from build123d import *

# Parameters (mm, degrees)
BOSS_EXTRUDE1_DEPTH     = 3
HOLE2_AT_2_COUNT        = 2
HOLE2_AT_2_PITCH        = 6
HOLE2_AT_3_COUNT        = 2
HOLE2_AT_3_PITCH        = 12
HOLE3_OUTLINE_R         = 2.5
HOLE3_DEPTH             = 1.5
SKETCH8_R               = 2.5
CUT_EXTRUDE1_DEPTH      = 1
FILL_START              = 2
FILL_PATTERN2_OUTLINE_R = 2.5
FILL_PATTERN2_DEPTH     = 1
HOLE6_D                 = 4
HOLE6_DEPTH             = 1.5
HOLE6_CBORE_D           = 5
HOLE6_CBORE_DEPTH       = 1
HOLE6_TIP               = 1.201721238
HOLE7_D                 = 4
HOLE7_DEPTH             = 3
HOLE7_CBORE_D           = 5
HOLE7_CBORE_DEPTH       = 1
HOLE7_TIP               = 1.201721238
HOLE8_D                 = 2
HOLE8_DEPTH             = 3
HOLE8_CBORE_D           = 3.8
HOLE8_CBORE_DEPTH       = 1.5
HOLE8_TIP               = 0.600860619


# Read off the part's stored shape, not the designer's step: Hole3, Fill Pattern2
with BuildPart() as part:
    # Sketch1 → Boss-Extrude1 (new body)
    with BuildSketch(Plane(origin=(0, 0, 0), x_dir=(1, 0, 0), z_dir=(0, 1, 0))):
        with BuildLine():
            Line((-12, 9), (12, 9))
            ThreePointArc((12, 9), (14.121320344, 8.121320344), (15, 6))
            Line((15, 6), (15, -6))
            ThreePointArc((15, -6), (14.121320344, -8.121320344), (12, -9))
            Line((12, -9), (-12, -9))
            ThreePointArc((-12, -9), (-14.121320344, -8.121320344), (-15, -6))
            Line((-15, -6), (-15, 6))
            ThreePointArc((-15, 6), (-14.121320344, 8.121320344), (-12, 9))
        make_face()
    extrude(amount=BOSS_EXTRUDE1_DEPTH)

    # Sketch3 → Hole2 (revolve, cut)
    with BuildSketch(Plane(origin=(-11.5, 3, -6), x_dir=(0, 0, 1), z_dir=(1, 0, 0))):
        Polygon((0, 0), (0, 2.701721238), (2, 1.5), (2, 0.8), (2.5, 0.8), (2.5, 0), align=None)
    hole2 = revolve(axis=Axis((-11.5, 14.310875039, -6), (0, -1, 0)), mode=Mode.SUBTRACT)

    # Hole2 at 2: Hole2 ×2
    with Locations(*[(0, 0, i * HOLE2_AT_2_PITCH) for i in range(1, HOLE2_AT_2_COUNT)]):
        add(hole2, mode=Mode.SUBTRACT)

    # Hole2 at 3: Hole2 ×2
    with Locations(*[(0, 0, i * HOLE2_AT_3_PITCH) for i in range(1, HOLE2_AT_3_COUNT)]):
        add(hole2, mode=Mode.SUBTRACT)

    # Hole3 outline → Hole3 (cut)
    with BuildSketch(Plane(origin=(0, 0, 0), x_dir=(1, 0, 0), z_dir=(0, 1, 0))):
        with Locations((-11.5, -6)):
            Circle(HOLE3_OUTLINE_R)
        with Locations((-11.5, 0)):
            Circle(HOLE3_OUTLINE_R)
        with Locations((-11.5, 6)):
            Circle(HOLE3_OUTLINE_R)
    hole3 = extrude(amount=HOLE3_DEPTH, mode=Mode.SUBTRACT)

    # Mirror1: Hole2, Hole3 across plane
    add(hole2.mirror(Plane(origin=(0, 0, 0), x_dir=(0, 0, 1), z_dir=(1, 0, 0))), mode=Mode.SUBTRACT)
    add(hole3.mirror(Plane(origin=(0, 0, 0), x_dir=(0, 0, 1), z_dir=(1, 0, 0))), mode=Mode.SUBTRACT)

    # Mirror1 copy 1 sketch → Mirror1 copy 1 (revolve, cut)
    with BuildSketch(Plane(origin=(11.5, 3, 0), x_dir=(0, 0, 1), z_dir=(-1, 0, 0))):
        Polygon((0, 0), (0, -2.701721238), (2, -1.5), (2, -0.8), (2.5, -0.8), (2.5, 0), align=None)
    revolve(axis=Axis((11.5, 14.310875039, 0), (0, 1, 0)), mode=Mode.SUBTRACT)

    # Mirror1 copy 2 sketch → Mirror1 copy 2 (revolve, cut)
    with BuildSketch(Plane(origin=(11.5, 3, 6), x_dir=(0, 0, 1), z_dir=(-1, 0, 0))):
        Polygon((0, 0), (0, -2.701721238), (2, -1.5), (2, -0.8), (2.5, -0.8), (2.5, 0), align=None)
    revolve(axis=Axis((11.5, 14.310875039, 6), (0, 1, 0)), mode=Mode.SUBTRACT)

    # Sketch8 → Cut-Extrude1 (cut)
    with BuildSketch(Plane(origin=(0, 3, 0), x_dir=(1, 0, 0), z_dir=(0, 1, 0))):
        with Locations(Location((0, 0, 0), (0, 0, 270))):
            Circle(SKETCH8_R)
    extrude(amount=-CUT_EXTRUDE1_DEPTH, mode=Mode.SUBTRACT)

    # Fill Pattern2 outline → Fill Pattern2 (cut)
    with BuildSketch(Plane(origin=(0, 0, 0), x_dir=(1, 0, 0), z_dir=(0, 1, 0)).offset(FILL_START)):
        with Locations((-6, -6)):
            Circle(FILL_PATTERN2_OUTLINE_R)
        with Locations((0, -6)):
            Circle(FILL_PATTERN2_OUTLINE_R)
        with Locations((6, -6)):
            Circle(FILL_PATTERN2_OUTLINE_R)
        with Locations((6, 0)):
            Circle(FILL_PATTERN2_OUTLINE_R)
        with Locations((6, 6)):
            Circle(FILL_PATTERN2_OUTLINE_R)
        with Locations((0, 6)):
            Circle(FILL_PATTERN2_OUTLINE_R)
        with Locations((-6, 6)):
            Circle(FILL_PATTERN2_OUTLINE_R)
        with Locations((-6, 0)):
            Circle(FILL_PATTERN2_OUTLINE_R)
    extrude(amount=FILL_PATTERN2_DEPTH, mode=Mode.SUBTRACT)

    # Hole6
    with Locations(Plane(origin=(0, 3, 0), x_dir=(1, 0, 0), z_dir=(0, 1, 0))):
        with Locations((0, 0)):
            CounterBoreHole(HOLE6_D / 2, HOLE6_CBORE_D / 2, HOLE6_CBORE_DEPTH, depth=HOLE6_DEPTH)
            with Locations((0, 0, -(HOLE6_DEPTH + HOLE6_TIP / 2))):  # 118° drill point
                Cone(0, HOLE6_D / 2, HOLE6_TIP, mode=Mode.SUBTRACT)

    # Hole7
    with Locations(Plane(origin=(0, 0, 0), x_dir=(-1, 0, 0), z_dir=(0, -1, 0))):
        with Locations((0, 0)):
            CounterBoreHole(HOLE7_D / 2, HOLE7_CBORE_D / 2, HOLE7_CBORE_DEPTH, depth=HOLE7_DEPTH)
            with Locations((0, 0, -(HOLE7_DEPTH + HOLE7_TIP / 2))):  # 118° drill point
                Cone(0, HOLE7_D / 2, HOLE7_TIP, mode=Mode.SUBTRACT)

    # Hole8
    with Locations(Plane(origin=(0, 3, 0), x_dir=(1, 0, 0), z_dir=(0, 1, 0))):
        with Locations((-5, -5), (-5, 5), (5, 5), (5, -5)):
            CounterBoreHole(HOLE8_D / 2, HOLE8_CBORE_D / 2, HOLE8_CBORE_DEPTH, depth=HOLE8_DEPTH)
            with Locations((0, 0, -(HOLE8_DEPTH + HOLE8_TIP / 2))):  # 118° drill point
                Cone(0, HOLE8_D / 2, HOLE8_TIP, mode=Mode.SUBTRACT)


solid = part.part
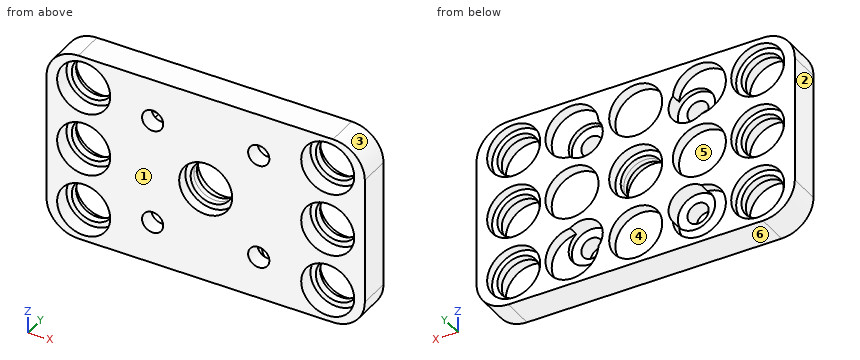
Read the model definition and answer for the solid it produces. Units are mm, in the model's axes. Face numbers are marked on the shaded views. A direction names the side the tool comes from. Give positions to 0.01 mm unless a question says otherwise; leave off trailing zeros. Write each loop counter-clockwise with the first axis right and the second up, starting at its lowest first coordinate (ties: lowest second). Pieces come first, ordered by that corner, then holes. Notation, with made-up numbers: (43, 23) -> (61, 23) arc R32 cw to (61, 49) -> close; hole circle Ø10 at (-14, 51). An arc over 180 degrees is marked (long way). Answer as a JSON object with one key per item and string values. Group by question number.
1) A tool of negligible diameter and unlimited length cuts with its end or side. For the marked faces 5 and 6, from which of +Z, -Z, +X, -X, +Y, -Y can it reach the whole face along a straight path? Write none if from no direction.
2) Find section A-A (y = 0.45). Count the separate pieces of the cut face and the enclosed holes in it, and give its area (3 significant figures).
3) Find section B-B (x = 0). Write down the section's boundary in (y, z), and give its area (3 significant figures).
4) Consider L1, parallel to Z at x = 0, y = 2.7; L2, parallel to Z at x = 3.75, y = 1.75; L3, parallel to X at y = 2.4, z = 6.25. Determine where each line is inside the solid, lowest interval first. Write a range as from..to.
5) The mould has two halves that part along X. Classify the marked faces 1, 2, 3 and 4: +X half, -X half, draft (parallel to the pull), parting line (faces both ways), or undercut.
6) Each of these flat-tipped pins is pushed along its axis until it touches: P1, Ø1.5, axis at x = -11.5, z = 5, coming from the +Y side; P2, Ø6, axis at x = 6, z = 6, coming from the -Y side; P3, Ø1.5, axis at x = 5, z = 0, coming from the +Y side; P4, Ø4.5, axis at x = 11.5, z = 6, coming from the +Y side. Where does it stop, or does it pass through?
Values follow:
{
 "1": {"face 5": "+Y", "face 6": "-Z, +X, -X, +Y, -Y"},
 "2": {"separate pieces": "1", "enclosed holes": "11", "area": "382 mm2"},
 "3": {"outline": "(0, -9) -> (3, -9) -> (3, -8.5) -> (2, -8.5) -> (2, -3.5) -> (3, -3.5) -> (3, -2.5) -> (2, -2.5) -> (2, -2) -> (1, -2) -> (1, -2.5) -> (0, -2.5) -> close; (0, 2.5) -> (1, 2.5) -> (1, 2) -> (2, 2) -> (2, 2.5) -> (3, 2.5) -> (3, 3.5) -> (2, 3.5) -> (2, 8.5) -> (3, 8.5) -> (3, 9) -> (0, 9) -> close", "area": "30.0 mm2"},
 "4": {"L1": "z = -9..-8.5, -3.5..-2.5, 2.5..3.5, 8.5..9", "L2": "z = -9..-6.43, -3.57..3.57, 6.43..9", "L3": "x = -14.99..-13.99, -9.01..-8.49, -3.51..-2.49, 2.49..3.51, 8.49..9.01, 13.99..14.99"},
 "5": {"face 1": "draft", "face 2": "-X half", "face 3": "+X half", "face 4": "undercut"},
 "6": {"P1": "passes through", "P2": "stops at y = 0", "P3": "stops at y = 2", "P4": "stops at y = 2.2"}
}
